```python
from build123d import *

# Parameters (mm, degrees)
SKETCH1_R           = 6
BOSS_EXTRUDE1_DEPTH = 1
FILLET2_R           = 0.5
SKETCH3_R           = 3
SKETCH3_R_2         = 2.5
BOSS_EXTRUDE2_DEPTH = 3.7
SKETCH4_R           = 2.5
CUT_EXTRUDE1_DEPTH  = 10.256889391
BOSS_EXTRUDE3_DEPTH = 3.7
SKETCH6_R           = 0.75
CUT_EXTRUDE2_DEPTH  = 10.256889391


with BuildPart() as part:
    # Sketch1 → Boss-Extrude1 (new body)
    with BuildSketch(Plane(origin=(0, 0, 0), x_dir=(0, 0, -1), z_dir=(1, 0, 0))):
        Circle(SKETCH1_R)
    extrude(amount=BOSS_EXTRUDE1_DEPTH)

    # Fillet2
    fillet2_edges = [part.edges().sort_by_distance(p)[0] for p in [
        (1, 0, 6),
    ]]
    fillet(fillet2_edges, radius=FILLET2_R)

    # Sketch3 → Boss-Extrude2 (add)
    with BuildSketch(Plane(origin=(1, 0, 0), x_dir=(0, 0, -1), z_dir=(1, 0, 0))):
        Circle(SKETCH3_R)
        Circle(SKETCH3_R_2, mode=Mode.SUBTRACT)
    extrude(amount=BOSS_EXTRUDE2_DEPTH)

    # Sketch4 → Cut-Extrude1 (cut, through all)
    with BuildSketch(Plane(origin=(1, 0, 0), x_dir=(0, 0, -1), z_dir=(1, 0, 0))):
        Circle(SKETCH4_R)
    extrude(amount=-CUT_EXTRUDE1_DEPTH, mode=Mode.SUBTRACT)

    # Sketch5 → Boss-Extrude3 (add, through all)
    with BuildSketch(Plane(origin=(1, 0, 0), x_dir=(0, 0, -1), z_dir=(1, 0, 0))):
        with BuildLine():
            Line((-2.537715508, 0.25), (-1.984313483, 0.25))
            ThreePointArc((-1.984313483, 0.25), (-1.931851653, 0.51763809), (-1.843465886, 0.775650391))
            Line((-1.843465886, 0.775650391), (-2.322726098, 1.052351403))
            ThreePointArc((-2.322726098, 1.052351403), (-2.463110857, 0.659988565), (-2.537715508, 0.25))
        make_face()
        with BuildLine():
            Line((-2.537715508, -0.25), (-1.984313483, -0.25))
            ThreePointArc((-1.984313483, -0.25), (-1.931851653, -0.51763809), (-1.843465886, -0.775650391))
            Line((-1.843465886, -0.775650391), (-2.322726098, -1.052351403))
            ThreePointArc((-2.322726098, -1.052351403), (-2.463110857, -0.659988565), (-2.537715508, -0.25))
        make_face()
        with BuildLine():
            Line((-2.072726098, 1.485364105), (-1.593465886, 1.208663093))
            ThreePointArc((-1.593465886, 1.208663093), (-1.414213562, 1.414213562), (-1.208663093, 1.593465886))
            Line((-1.208663093, 1.593465886), (-1.485364105, 2.072726098))
            ThreePointArc((-1.485364105, 2.072726098), (-1.803122292, 1.803122292), (-2.072726098, 1.485364105))
        make_face()
        with BuildLine():
            Line((-1.052351403, 2.322726098), (-0.775650391, 1.843465886))
            ThreePointArc((-0.775650391, 1.843465886), (-0.51763809, 1.931851653), (-0.25, 1.984313483))
            Line((-0.25, 1.984313483), (-0.25, 2.537715508))
            ThreePointArc((-0.25, 2.537715508), (-0.659988565, 2.463110857), (-1.052351403, 2.322726098))
        make_face()
        with BuildLine():
            Line((0.25, 2.537715508), (0.25, 1.984313483))
            ThreePointArc((0.25, 1.984313483), (0.51763809, 1.931851653), (0.775650391, 1.843465886))
            Line((0.775650391, 1.843465886), (1.052351403, 2.322726098))
            ThreePointArc((1.052351403, 2.322726098), (0.659988565, 2.463110857), (0.25, 2.537715508))
        make_face()
        with BuildLine():
            Line((1.485364105, 2.072726098), (1.208663093, 1.593465886))
            ThreePointArc((1.208663093, 1.593465886), (1.414213562, 1.414213562), (1.593465886, 1.208663093))
            Line((1.593465886, 1.208663093), (2.072726098, 1.485364105))
            ThreePointArc((2.072726098, 1.485364105), (1.803122292, 1.803122292), (1.485364105, 2.072726098))
        make_face()
        with BuildLine():
            Line((2.322726098, 1.052351403), (1.843465886, 0.775650391))
            ThreePointArc((1.843465886, 0.775650391), (1.931851653, 0.51763809), (1.984313483, 0.25))
            Line((1.984313483, 0.25), (2.537715508, 0.25))
            ThreePointArc((2.537715508, 0.25), (2.463110857, 0.659988565), (2.322726098, 1.052351403))
        make_face()
        with BuildLine():
            Line((2.537715508, -0.25), (1.984313483, -0.25))
            ThreePointArc((1.984313483, -0.25), (1.931851653, -0.51763809), (1.843465886, -0.775650391))
            Line((1.843465886, -0.775650391), (2.322726098, -1.052351403))
            ThreePointArc((2.322726098, -1.052351403), (2.463110857, -0.659988565), (2.537715508, -0.25))
        make_face()
        with BuildLine():
            Line((2.072726098, -1.485364105), (1.593465886, -1.208663093))
            ThreePointArc((1.593465886, -1.208663093), (1.414213562, -1.414213562), (1.208663093, -1.593465886))
            Line((1.208663093, -1.593465886), (1.485364105, -2.072726098))
            ThreePointArc((1.485364105, -2.072726098), (1.803122292, -1.803122292), (2.072726098, -1.485364105))
        make_face()
        with BuildLine():
            Line((1.052351403, -2.322726098), (0.775650391, -1.843465886))
            ThreePointArc((0.775650391, -1.843465886), (0.51763809, -1.931851653), (0.25, -1.984313483))
            Line((0.25, -1.984313483), (0.25, -2.537715508))
            ThreePointArc((0.25, -2.537715508), (0.659988565, -2.463110857), (1.052351403, -2.322726098))
        make_face()
        with BuildLine():
            Line((-0.25, -2.537715508), (-0.25, -1.984313483))
            ThreePointArc((-0.25, -1.984313483), (-0.51763809, -1.931851653), (-0.775650391, -1.843465886))
            Line((-0.775650391, -1.843465886), (-1.052351403, -2.322726098))
            ThreePointArc((-1.052351403, -2.322726098), (-0.659988565, -2.463110857), (-0.25, -2.537715508))
        make_face()
        with BuildLine():
            Line((-1.485364105, -2.072726098), (-1.208663093, -1.593465886))
            ThreePointArc((-1.208663093, -1.593465886), (-1.414213562, -1.414213562), (-1.593465886, -1.208663093))
            Line((-1.593465886, -1.208663093), (-2.072726098, -1.485364105))
            ThreePointArc((-2.072726098, -1.485364105), (-1.803122292, -1.803122292), (-1.485364105, -2.072726098))
        make_face()
    extrude(amount=BOSS_EXTRUDE3_DEPTH)

    # Sketch6 → Cut-Extrude2 (cut, through all)
    with BuildSketch(Plane(origin=(1, 0, 0), x_dir=(0, 0, -1), z_dir=(1, 0, 0))):
        with Locations((-4.25, 0)):
            Circle(SKETCH6_R)
        with Locations((0, 4.25)):
            Circle(SKETCH6_R)
        with Locations((4.25, 0)):
            Circle(SKETCH6_R)
        with Locations((0, -4.25)):
            Circle(SKETCH6_R)
    extrude(amount=-CUT_EXTRUDE2_DEPTH, mode=Mode.SUBTRACT)


solid = part.part
```
Geometry: final body of the model. Coordinates: model frame, mm. A direction names the side the tool comes from. Round coordinates to 2 decimals unless told otherwise and drop trailing zeros. Write each loop counter-clockwise with the first axis right and the second up, starting at its lowest first coordinate (ties: lowest second). Pieces come first, ordered by that corner, then holes.
Item 1: Set-up query: faces 1 (the face through (1, -1.6, 1.6)), 2 (the face through (0.5, 0, 5)). Return all of +Z, -Z, +X, -X, +Y, -Y with unobstructed straight access to the full face (end or side cutting, diameter ignored); none if empty.
Item 2: Material intervals for L1, parallel to Y at x = 0.5, z = 0; L2, parallel to X at y = -3.25, z = 0.25; L3, parallel to Y at x = 0.9, z = 0.5, sorted ascending.
Item 3: Mould query, pull axis Z, two halves, no side actions, for faces 3 (the face through (3, 0, 3)), 4 (the face through (1, -2.4, -2.4)), 5 (the face through (1, 1.6, -1.6)). Classes: +Z half, -Z half, draft (parallel to the pull), parting line (faces both ways), or undercut.
Item 4: Section query A-A (z = 0). Return loops of the section in (x, y), plus the area to 3 significant figures.
Item 5: Pin query (flat end, axial travel): P1, Ø2, axis at y = -4.5, z = -3.5, coming from the +X side; P2, Ø0.5, axis at y = 0.5, z = 2, coming from the -X side; P3, Ø2, axis at x = 3, y = 3, coming from the -Z side. Return the tip coordinate at first contact, or that it passes through.
Completed:
1. face 1: -X
1. face 2: +X, -X
2. L1: y = -6 to -5, -3.5 to -2.5, 2.5 to 3.5, 5 to 6
2. L2: x = 0 to 1
2. L3: y = -5.78 to -4.81, -3.69 to -2.45, 2.45 to 3.69, 4.81 to 5.78
3. face 3: parting line
3. face 4: draft
3. face 5: undercut
4. outline: (0, -6) - (0.5, -6) arc R0.5 ccw to (1, -5.5) - (1, -5) - (0, -5) - close; (0, -3.5) - (1, -3.5) - (1, -3) - (4.7, -3) - (4.7, -2.5) - (0, -2.5) - close; (0, 2.5) - (4.7, 2.5) - (4.7, 3) - (1, 3) - (1, 3.5) - (0, 3.5) - close; (0, 5) - (1, 5) - (1, 5.5) arc R0.5 ccw to (0.5, 6) - (0, 6) - close
4. area: 7.59 mm2
5. P1: stops at x = 1
5. P2: stops at x = 1
5. P3: stops at z = -2.24
